Autodesk Inventor part; units mm, degrees
ref_plane "YZ Plane" through (0, 0, 0) normal (1, 0, 0) x (0, 1, 0)
ref_plane "XZ Plane" through (0, 0, 0) normal (0, 1, 0) x (-1, 0, 0)
ref_plane "XY Plane" through (0, 0, 0) normal (0, 0, 1) x (1, 0, 0)
sketch "Sketch1" plane through (0, 0, 0) normal (0, 1, 0) x (-1, 0, 0)
  circle A0 centre (0, 0) radius 17.325
  circle A1 centre (0, 0) radius 7.325
  dimension "d0" = 34.65
  dimension "d1" = 14.65
extrude "Extrusion1" add sketch "Sketch1" along normal blind 2
sketch "Sketch2" plane through (0, 2, 0) normal (0, 1, 0) x (1, 0, 0)
  line L0 (-22.325, -1) -> (-12.325, -1)
  line L1 (-12.325, -1) -> (-12.325, 1)
  line L2 (-12.325, 1) -> (-22.325, 1)
  line L3 (-22.325, 1) -> (-22.325, -1)
  point P0 (0, 0)
  dimension "d4" = 1
  dimension "d5" = 2
  dimension "d6" = 12.325
  dimension "d7" = 10
extrude "Extrusion2" cut sketch "Sketch2" against normal blind 2
pattern_circular "Circular Pattern2" count 6 over 360 about axis through (0, -10, 0) along (0, 1, 0) of "Extrusion2"
properties part number "Ring_n7"
Verification items for the finished model (mm, model axes). A direction names the side the tool comes from. Coordinates: 2 decimals unless noted, no trailing zeros. Loops run counter-clockwise (first coordinate to the right, second up) from the corner with the lowest first, then second, coordinate; pieces in that order, holes last. Notation, with made-up numbers: (49, -24) -> (106, -24) arc R31 ccw to (106, 3) -> close; hole circle Ø5 at (26.25, 73). An arc over 180 degrees is marked (long way). Write each question's results on one line, items separated by ' | '.
Item 1: Tool access check on faces 4 (the face through (15, 1, -1)), 5 (the face through (8.254, 1.014, -12.296)), 6 (the face through (0.2, 0, -7.5)), 7 (the face through (-15, 1, 1)). Record the directions out of +Z, -Z, +X, -X, +Y, -Y that give a thin tool (end or side, any length) a straight path to the whole face; none if there is none.
Found:
face 4: +X, +Y, -Y | face 5: +Y, -Y | face 6: +Z, -Z, +X, -X, -Y | face 7: -X, +Y, -Y
Item 2: Section check A-A, the plane x = 0. Enter the section's corners in (y, z) (3 decimals).
Found:
outline: (0, -17.325) -> (2, -17.325) -> (2, -7.325) -> (0, -7.325) -> close; (0, 7.325) -> (2, 7.325) -> (2, 17.325) -> (0, 17.325) -> close
Item 3: Section check C-C, the plane y = 0.8. Enter the section's corners in (x, z) (3 decimals).
Found:
outline: (-17.296, -1) arc R17.325 ccw to (-9.514, -14.479) -> (-7.029, -10.174) -> (-5.296, -11.174) -> (-7.782, -15.479) arc R17.325 ccw to (7.782, -15.479) -> (5.296, -11.174) -> (7.029, -10.174) -> (9.514, -14.479) arc R17.325 ccw to (17.296, -1) -> (12.325, -1) -> (12.325, 1) -> (17.296, 1) arc R17.325 ccw to (9.514, 14.479) -> (7.029, 10.174) -> (5.296, 11.174) -> (7.782, 15.479) arc R17.325 ccw to (-7.782, 15.479) -> (-5.296, 11.174) -> (-7.029, 10.174) -> (-9.514, 14.479) arc R17.325 ccw to (-17.296, 1) -> (-12.325, 1) -> (-12.325, -1) -> close; hole circle Ø14.65 at (0, 0)
Item 4: Mould release check, pull along X, two halves, no side actions. Record for faces 1 (the face through (8.29, 1.01, 12.36)), 2 (the face through (14.947, 0.986, -8.76)), 3 (the face through (0.113, 0.986, 17.325)): +X half, -X half, draft (parallel to the pull), parting line (faces both ways), or undercut.
Found:
face 1: undercut | face 2: +X half | face 3: parting line
Item 5: Gauge pin test, flat end, axial feed: pin 1 (1 mm diameter, centred on x = -12.5, y = 0.5, fed in from -Z). Record the tip position at first contact, or that the pin passes through.
Found:
pin 1: stops at z = -12.5
Item 6: Section check B-B, the plane z = 0. Enter the section's corners in (x, y) (3 decimals), plus the area to 3 significant figures.
Found:
outline: (-12.325, 0) -> (-7.325, 0) -> (-7.325, 2) -> (-12.325, 2) -> close; (7.325, 0) -> (12.325, 0) -> (12.325, 2) -> (7.325, 2) -> close | area: 20.0 mm2
Item 7: Material ranges on L1, parallel to Z at x = -5.5, y = 0.9; L2, parallel to Z at x = 6.5, y = 1.4; L3, parallel to X at y = 1.35, z = -11.5, recorded low to high.
Found:
L1: z = -16.43 to -11.53, -11.06 to -4.84, 4.84 to 11.06, 11.53 to 16.43 | L2: z = -16.06 to -13.26, -10.48 to -3.38, 3.38 to 10.48, 13.26 to 16.06 | L3: x = -12.96 to -7.79, -5.48 to 5.48, 7.79 to 12.96
Item 8: Section check D-D, the plane x = 11. Enter the section's corners in (y, z), plus the area to 3 significant figures.
Found:
outline: (0, -13.38) -> (2, -13.38) -> (2, 13.38) -> (0, 13.38) -> close | area: 53.5 mm2
